Part print with two shaded views. Sizes in mm from the minimum x, y, z corner. A direction names the side the tool comes from. Give positions to 0.01 mm unless a question says otherwise; leave off trailing zeros. Order: outer loops, then holes, each group sorted by start corner. A loop starts at its lowest first (then second) coordinate and runs counter-clockwise, first axis right, second up. Notation, with made-up numbers: M -34.75,-34.5 L -25.75,-34.5 A15 ccw -25.75,-28.5 Z; hole C 80,82 d2. An arc over 180 degrees is marked long. Return JSON: item names as keys, results as strings. Group by question number.
1. Wall check: probe 1 along X at (y, z) = (27.5, 18); probe 2 along X at (y, z) = (46.5, 36); probe 3 along Y at (x, z) = (47, 31.5). Give the ranges that are in metal, low to high. Write a range as [from, to].
2. Slice it at A-A on z = 4.5. List the corners of the cut face in (x, y), then the cut area to 3 significant figures.
3. Two-plate mould, pull along X, no slides. Class the marked faces 5, 6, 7 and 8: released by +X, released by -X, zero draft, split by the parting line, or undercut.
4. Slice it at B-B on x = 55. List the corners of the cut face in (y, z).
5. Slice it at C-C on y = 43.5. List the corners of the cut face in (x, z).
6. Pin check, flat tips, straight feed: pin 1 (2 mm diameter, centred on x = 47, y = 25, fed in from +Z); pin 2 (4 mm diameter, centred on x = 40, y = 45, fed in from +Z); pin 3 (21.5 mm diameter, centred on x = 28.5, z = 30, fed in from -Y). Stop position of each tip, or through.
7. Slice it at D-D on z = 11. List the corners of the cut face in (x, y).
8. 3-axis set-ups, long thin cutter, end or side, ignore diameter. For the marked faces 1, 2, 3 and 4: which of +Z, -Z, +X, -X, +Y, -Y reach the whole face in a straight line?
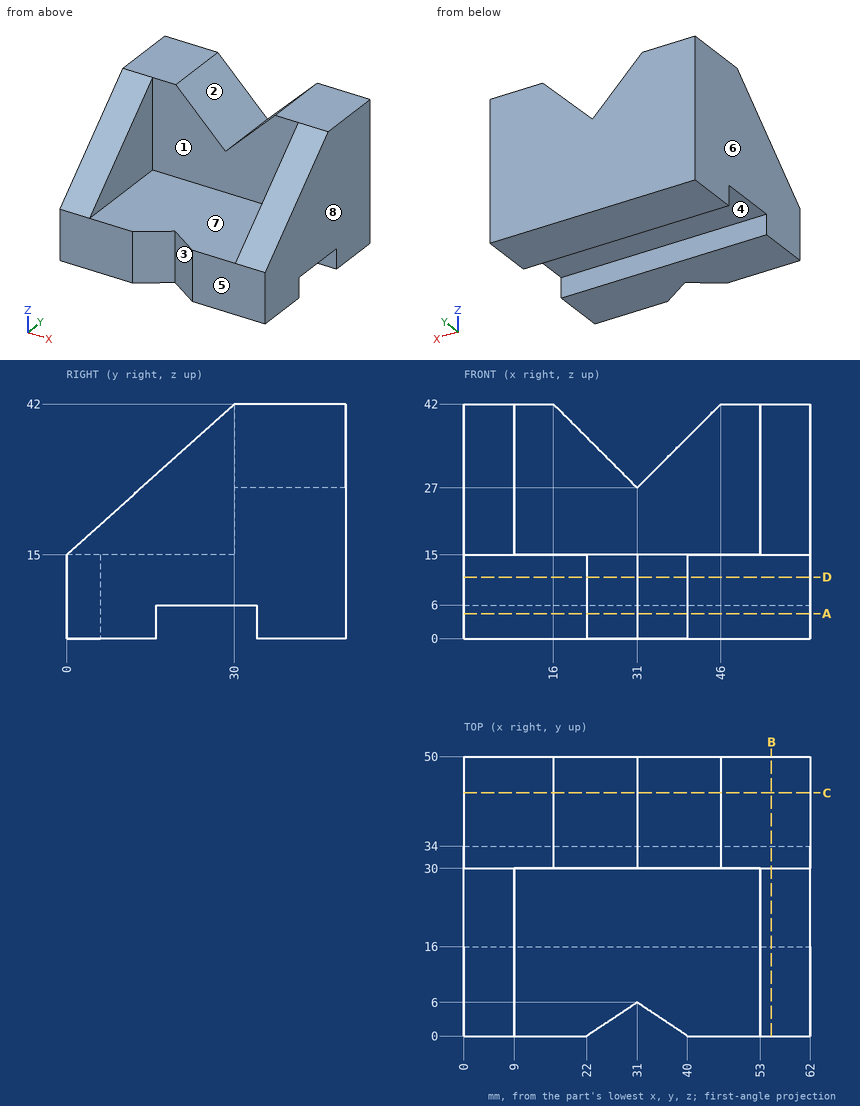
Result:
{
 "1": {"probe 1": "x = [0, 9], [53, 62]", "probe 2": "x = [0, 22], [40, 62]", "probe 3": "y = [30, 50]"},
 "2": {"outline": "M 0,0 L 22,0 L 31,6 L 40,0 L 62,0 L 62,16 L 0,16 Z; M 0,34 L 62,34 L 62,50 L 0,50 Z", "area": "1,930 mm2"},
 "3": {"face 5": "zero draft", "face 6": "released by -X", "face 7": "undercut", "face 8": "released by +X"},
 "4": {"outline": "M 0,0 L 16,0 L 16,6 L 34,6 L 34,0 L 50,0 L 50,42 L 30,42 L 0,15 Z"},
 "5": {"outline": "M 0,0 L 62,0 L 62,42 L 46,42 L 31,27 L 16,42 L 0,42 Z"},
 "6": {"pin 1": "stops at z = 15", "pin 2": "stops at z = 38", "pin 3": "stops at y = 30"},
 "7": {"outline": "M 0,0 L 22,0 L 31,6 L 40,0 L 62,0 L 62,50 L 0,50 Z"},
 "8": {"face 1": "+Z, -Y", "face 2": "+Z, +Y, -Y", "face 3": "+Z, -Z, -Y", "face 4": "-Z, +X, -X"}
}
